Geometry: final body of the model. Coordinates: model frame, mm. A direction names the side the tool comes from. Give positions to 0.01 mm unless a question says otherwise; leave off trailing zeros. Write each loop counter-clockwise with the first axis right and the second up, starting at its lowest first coordinate (ties: lowest second). Pieces come first, ordered by that corner, then holes. Notation, with made-up numbers: M -26,67 L 13,67 A16 ccw 13,95 Z; hole C 61.5,28 d11. An arc over 180 degrees is marked long. Answer as a JSON object with one key per item and string values.
from build123d import *

# Parameters (mm, degrees)
SKETCH_1_R          = 12.5
EXTRUDE_1_DEPTH     = 1
SKETCH_5_R          = 4
EXTRUDE_4_DEPTH     = 2
SKETCH_6_R          = 12.5
EXTRUDE_5_DEPTH     = 1
SKETCH_7_R          = 4
EXTRUDE_6_DEPTH     = 2
SKETCH_8_R          = 12.5
EXTRUDE_7_DEPTH     = 1
SKETCH_9_R          = 4
EXTRUDE_8_DEPTH     = 2
SKETCH_10_R         = 12.5
EXTRUDE_9_DEPTH     = 1
SKETCH_11_R         = 4
EXTRUDE_10_DEPTH    = 2
SKETCH_12_R         = 12.5
EXTRUDE_11_DEPTH    = 1
SKETCH_13_R         = 4
EXTRUDE_12_DEPTH    = 2
SKETCH_14_R         = 12.5
EXTRUDE_13_DEPTH    = 1
SKETCH_15_R         = 4
EXTRUDE_14_DEPTH    = 2
SKETCH_16_R         = 12.5
EXTRUDE_15_DEPTH    = 1
SKETCH_17_R         = 4
EXTRUDE_16_DEPTH    = 2
SKETCH_18_R         = 12.5
EXTRUDE_17_DEPTH    = 1
SKETCH_19_R         = 4
EXTRUDE_18_DEPTH    = 2
SKETCH_20_R         = 12.5
EXTRUDE_19_DEPTH    = 1
SKETCH_21_R         = 4
EXTRUDE_20_DEPTH    = 2
SKETCH_22_R         = 12.5
EXTRUDE_21_DEPTH    = 1
SKETCH_23_R         = 4
EXTRUDE_22_DEPTH    = 2
SKETCH_24_R         = 12.5
EXTRUDE_23_DEPTH    = 1
SKETCH_25_R         = 4
EXTRUDE_24_DEPTH    = 2
SKETCH_26_R         = 9
EXTRUDE_25_DEPTH    = 1
SKETCH_27_R         = 4
EXTRUDE_26_DEPTH    = 2
SKETCH_28_R         = 9
EXTRUDE_27_DEPTH    = 2
SKETCH_29_R         = 7
EXTRUDE_28_DEPTH    = 5
SKETCH_30_R         = 9
EXTRUDE_29_DEPTH    = 3
SKETCH_31_R         = 3
CUT_EXTRUDE_1_DEPTH = 50.279813311


with BuildPart() as part:
    # 草图1 → 凸台-拉伸1 (new body)
    with BuildSketch(Plane(origin=(0, 0, 0), x_dir=(1, 0, 0), z_dir=(0, 1, 0))):
        with Locations(Location((0, 0, 0), (0, 0, 270))):
            Circle(SKETCH_1_R)
    extrude(amount=EXTRUDE_1_DEPTH)

    # 草图5 → 凸台-拉伸4 (add)
    with BuildSketch(Plane(origin=(0, 1, 0), x_dir=(1, 0, 0), z_dir=(0, 1, 0))):
        with Locations(Location((0, 0, 0), (0, 0, 270))):
            Circle(SKETCH_5_R)
    extrude(amount=EXTRUDE_4_DEPTH)

    # 草图6 → 凸台-拉伸5 (add)
    with BuildSketch(Plane(origin=(0, 3, 0), x_dir=(1, 0, 0), z_dir=(0, 1, 0))):
        with Locations(Location((0, 0, 0), (0, 0, 270))):
            Circle(SKETCH_6_R)
    extrude(amount=EXTRUDE_5_DEPTH)

    # 草图7 → 凸台-拉伸6 (add)
    with BuildSketch(Plane(origin=(0, 4, 0), x_dir=(1, 0, 0), z_dir=(0, 1, 0))):
        with Locations(Location((0, 0, 0), (0, 0, 270))):
            Circle(SKETCH_7_R)
    extrude(amount=EXTRUDE_6_DEPTH)

    # 草图8 → 凸台-拉伸7 (add)
    with BuildSketch(Plane(origin=(0, 6, 0), x_dir=(1, 0, 0), z_dir=(0, 1, 0))):
        with Locations(Location((0, 0, 0), (0, 0, 270))):
            Circle(SKETCH_8_R)
    extrude(amount=EXTRUDE_7_DEPTH)

    # 草图9 → 凸台-拉伸8 (add)
    with BuildSketch(Plane(origin=(0, 7, 0), x_dir=(1, 0, 0), z_dir=(0, 1, 0))):
        with Locations(Location((0, 0, 0), (0, 0, 270))):
            Circle(SKETCH_9_R)
    extrude(amount=EXTRUDE_8_DEPTH)

    # 草图10 → 凸台-拉伸9 (add)
    with BuildSketch(Plane(origin=(0, 9, 0), x_dir=(1, 0, 0), z_dir=(0, 1, 0))):
        with Locations(Location((0, 0, 0), (0, 0, 270))):
            Circle(SKETCH_10_R)
    extrude(amount=EXTRUDE_9_DEPTH)

    # 草图11 → 凸台-拉伸10 (add)
    with BuildSketch(Plane(origin=(0, 10, 0), x_dir=(1, 0, 0), z_dir=(0, 1, 0))):
        with Locations(Location((0, 0, 0), (0, 0, 270))):
            Circle(SKETCH_11_R)
    extrude(amount=EXTRUDE_10_DEPTH)

    # 草图12 → 凸台-拉伸11 (add)
    with BuildSketch(Plane(origin=(0, 12, 0), x_dir=(1, 0, 0), z_dir=(0, 1, 0))):
        with Locations(Location((0, 0, 0), (0, 0, 270))):
            Circle(SKETCH_12_R)
    extrude(amount=EXTRUDE_11_DEPTH)

    # 草图13 → 凸台-拉伸12 (add)
    with BuildSketch(Plane(origin=(0, 13, 0), x_dir=(1, 0, 0), z_dir=(0, 1, 0))):
        with Locations(Location((0, 0, 0), (0, 0, 270))):
            Circle(SKETCH_13_R)
    extrude(amount=EXTRUDE_12_DEPTH)

    # 草图14 → 凸台-拉伸13 (add)
    with BuildSketch(Plane(origin=(0, 15, 0), x_dir=(1, 0, 0), z_dir=(0, 1, 0))):
        with Locations(Location((0, 0, 0), (0, 0, 270))):
            Circle(SKETCH_14_R)
    extrude(amount=EXTRUDE_13_DEPTH)

    # 草图15 → 凸台-拉伸14 (add)
    with BuildSketch(Plane(origin=(0, 16, 0), x_dir=(1, 0, 0), z_dir=(0, 1, 0))):
        with Locations(Location((0, 0, 0), (0, 0, 270))):
            Circle(SKETCH_15_R)
    extrude(amount=EXTRUDE_14_DEPTH)

    # 草图16 → 凸台-拉伸15 (add)
    with BuildSketch(Plane(origin=(0, 18, 0), x_dir=(1, 0, 0), z_dir=(0, 1, 0))):
        with Locations(Location((0, 0, 0), (0, 0, 270))):
            Circle(SKETCH_16_R)
    extrude(amount=EXTRUDE_15_DEPTH)

    # 草图17 → 凸台-拉伸16 (add)
    with BuildSketch(Plane(origin=(0, 19, 0), x_dir=(1, 0, 0), z_dir=(0, 1, 0))):
        with Locations(Location((0, 0, 0), (0, 0, 270))):
            Circle(SKETCH_17_R)
    extrude(amount=EXTRUDE_16_DEPTH)

    # 草图18 → 凸台-拉伸17 (add)
    with BuildSketch(Plane(origin=(0, 21, 0), x_dir=(1, 0, 0), z_dir=(0, 1, 0))):
        with Locations(Location((0, 0, 0), (0, 0, 270))):
            Circle(SKETCH_18_R)
    extrude(amount=EXTRUDE_17_DEPTH)

    # 草图19 → 凸台-拉伸18 (add)
    with BuildSketch(Plane(origin=(0, 22, 0), x_dir=(1, 0, 0), z_dir=(0, 1, 0))):
        with Locations(Location((0, 0, 0), (0, 0, 270))):
            Circle(SKETCH_19_R)
    extrude(amount=EXTRUDE_18_DEPTH)

    # 草图20 → 凸台-拉伸19 (add)
    with BuildSketch(Plane(origin=(0, 24, 0), x_dir=(1, 0, 0), z_dir=(0, 1, 0))):
        with Locations(Location((0, 0, 0), (0, 0, 270))):
            Circle(SKETCH_20_R)
    extrude(amount=EXTRUDE_19_DEPTH)

    # 草图21 → 凸台-拉伸20 (add)
    with BuildSketch(Plane(origin=(0, 25, 0), x_dir=(1, 0, 0), z_dir=(0, 1, 0))):
        with Locations(Location((0, 0, 0), (0, 0, 270))):
            Circle(SKETCH_21_R)
    extrude(amount=EXTRUDE_20_DEPTH)

    # 草图22 → 凸台-拉伸21 (add)
    with BuildSketch(Plane(origin=(0, 27, 0), x_dir=(1, 0, 0), z_dir=(0, 1, 0))):
        with Locations(Location((0, 0, 0), (0, 0, 270))):
            Circle(SKETCH_22_R)
    extrude(amount=EXTRUDE_21_DEPTH)

    # 草图23 → 凸台-拉伸22 (add)
    with BuildSketch(Plane(origin=(0, 28, 0), x_dir=(1, 0, 0), z_dir=(0, 1, 0))):
        with Locations(Location((0, 0, 0), (0, 0, 270))):
            Circle(SKETCH_23_R)
    extrude(amount=EXTRUDE_22_DEPTH)

    # 草图24 → 凸台-拉伸23 (add)
    with BuildSketch(Plane(origin=(0, 30, 0), x_dir=(1, 0, 0), z_dir=(0, 1, 0))):
        with Locations(Location((0, 0, 0), (0, 0, 270))):
            Circle(SKETCH_24_R)
    extrude(amount=EXTRUDE_23_DEPTH)

    # 草图25 → 凸台-拉伸24 (add)
    with BuildSketch(Plane(origin=(0, 31, 0), x_dir=(1, 0, 0), z_dir=(0, 1, 0))):
        with Locations(Location((0, 0, 0), (0, 0, 270))):
            Circle(SKETCH_25_R)
    extrude(amount=EXTRUDE_24_DEPTH)

    # 草图26 → 凸台-拉伸25 (add)
    with BuildSketch(Plane(origin=(0, 33, 0), x_dir=(1, 0, 0), z_dir=(0, 1, 0))):
        with Locations(Location((0, 0, 0), (0, 0, 270))):
            Circle(SKETCH_26_R)
    extrude(amount=EXTRUDE_25_DEPTH)

    # 草图27 → 凸台-拉伸26 (add)
    with BuildSketch(Plane(origin=(0, 34, 0), x_dir=(1, 0, 0), z_dir=(0, 1, 0))):
        with Locations(Location((0, 0, 0), (0, 0, 270))):
            Circle(SKETCH_27_R)
    extrude(amount=EXTRUDE_26_DEPTH)

    # 草图28 → 凸台-拉伸27 (add)
    with BuildSketch(Plane(origin=(0, 36, 0), x_dir=(1, 0, 0), z_dir=(0, 1, 0))):
        with Locations(Location((0, 0, 0), (0, 0, 270))):
            Circle(SKETCH_28_R)
    extrude(amount=EXTRUDE_27_DEPTH)

    # 草图29 → 凸台-拉伸28 (add)
    with BuildSketch(Plane(origin=(0, 38, 0), x_dir=(1, 0, 0), z_dir=(0, 1, 0))):
        with Locations(Location((0, 0, 0), (0, 0, 270))):
            Circle(SKETCH_29_R)
    extrude(amount=EXTRUDE_28_DEPTH)

    # 草图30 → 凸台-拉伸29 (add)
    with BuildSketch(Plane(origin=(0, 43, 0), x_dir=(1, 0, 0), z_dir=(0, 1, 0))):
        with Locations(Location((0, 0, 0), (0, 0, 270))):
            Circle(SKETCH_30_R)
    extrude(amount=EXTRUDE_29_DEPTH)

    # 草图31 → 切除-拉伸1 (cut, through all)
    with BuildSketch(Plane(origin=(0, 0, 0), x_dir=(-1, 0, 0), z_dir=(0, -1, 0))):
        with Locations(Location((0, 0, 0), (0, 0, 90))):
            Circle(SKETCH_31_R)
    extrude(amount=-CUT_EXTRUDE_1_DEPTH, mode=Mode.SUBTRACT)


solid = part.part
1) Contact query for flat-ended pins moving along their axis: P1, Ø2, axis at x = -4.5, y = 33.5, coming from the -Z side; P2, Ø8, axis at y = 14.5, z = -5, coming from the +X side; P3, Ø5, axis at x = 8, y = 8, coming from the -Z side. Output: stop coordinate, or through.
Geometry check:
{"P1": "stops at z = -8.29", "P2": "stops at x = 12.46", "P3": "stops at z = -11.12"}
2) Cut plane A-A on y = 32. Return loops of the section in (x, z).
Geometry check:
{"outline": "C 0,0 d8; hole C 0,0 d6"}
3) Cut plane B-B on x = 9.5. Give the number of separate pieces and of enclosed holes in the cut face, and give its area (3 significant figures).
Geometry check:
{"separate pieces": "11", "enclosed holes": "0", "area": "179 mm2"}
4) Line query: line 1 (X direction, y = 17, z = 0); line 2 (X direction, y = 33.5, z = -2.25); line 3 (Z direction, x = -4.75, y = 37). Output: solid intervals per line, ascending. Write a range as from..to.
Geometry check:
{"line 1": "x = -4..-3, 3..4", "line 2": "x = -8.71..-1.98, 1.98..8.71", "line 3": "z = -7.64..7.64"}
5) Cut plane D-D on y = 40.5. Return loops of the section in (x, z), and give its area (3 significant figures).
Geometry check:
{"outline": "C 0,0 d14; hole C 0,0 d6", "area": "126 mm2"}
6) Set-up query: faces 1 (the cylindrical face through (2.703, 36.986, 8.584)), 2 (the cylindrical face through (3.755, 6.493, 11.923)), 3 (the flat face through (3, 28, -3)). Return all of +Z, -Z, +X, -X, +Y, -Y with unobstructed straight access to the full face (end or side cutting, diameter ignored); none if empty.
Geometry check:
{"face 1": "+Y", "face 2": "+Y, -Y", "face 3": "none"}
